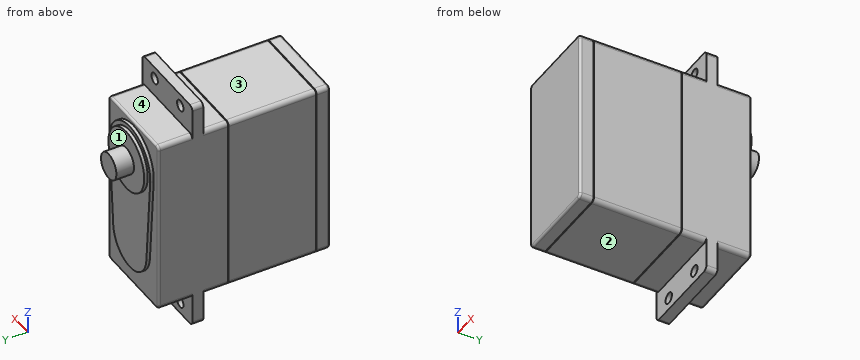
```python
from build123d import *

# Parameters (mm, degrees)
BOSS_EXTRU_1_DEPTH        = 9.75
BOSS_EXTRU_1_DEPTH_BACK   = 9.75
ESQUISSE1_W               = 40.5
ESQUISSE1_H               = 39
BOSS_EXTRU_2_DEPTH        = 0.8
CONG_6_R                  = 1
CONG_3_R                  = 0.5
ENL_V_MAT_EXTRU_3_DEPTH   = 0.2
ENL_V_MAT_EXTRU_2_DEPTH   = 0.2
BOSS_EXTRU_3_DEPTH        = 1.25
ENL_V_MAT_EXTRU_4_REACH   = 44.593
ESQUISSE10_R              = 1.25
SYM_TRIE3_COPY_1_REACH    = 44.593
SYM_TRIE3_COPY_1_SKETCH_R = 1.25


with BuildPart() as part:
    # Esquisse1 → Boss.-Extru.1 (new, two sides: drawn at the far end of the back side and taken through both)
    with BuildSketch(Plane(origin=(0, 0, 0), x_dir=(0, 0, -1), z_dir=(1, 0, 0)).offset(-BOSS_EXTRU_1_DEPTH_BACK)):
        Rectangle(ESQUISSE1_W, ESQUISSE1_H)
    extrude(amount=BOSS_EXTRU_1_DEPTH + BOSS_EXTRU_1_DEPTH_BACK)

    # Esquisse2 → Boss.-Extru.2 (add)
    with BuildSketch(Plane(origin=(13.65, 19.5, 0), x_dir=(0, 0, -1), z_dir=(0, 1, 0))):
        with BuildLine():
            Line((9.725609756, 20.13257629), (-10.664634146, 21.628555434))
            ThreePointArc((-10.664634146, 21.628555434), (-19.25, 13.65), (-10.664634146, 5.671444566))
            Line((-10.664634146, 5.671444566), (9.725609756, 7.16742371))
            ThreePointArc((9.725609756, 7.16742371), (15.75, 13.65), (9.725609756, 20.13257629))
        make_face()
    extrude(amount=BOSS_EXTRU_2_DEPTH)

    # Esquisse3 → R_volution1 (revolve)
    with BuildSketch(Plane(origin=(0, 0, 0), x_dir=(0, 0, -1), z_dir=(1, 0, 0)), mode=Mode.PRIVATE) as r_volution1_sk:
        Polygon((-4.25, 20.3), (-4.25, 21.1), (-8.25, 21.1), (-8.25, 25.1), (-11.25, 25.1), (-11.25, 20.3), align=None)
    revolve(r_volution1_sk.sketch.rotate(Axis((0, 19.890028941, 11.25), (0, -1, 0)), 180), axis=Axis((0, 19.890028941, 11.25), (0, -1, 0)))

    # Cong_6
    cong_6_edges = [part.edges().sort_by_distance(p)[0] for p in [
        (9.75, 0, 20.25),
        (-9.75, 0, -20.25),
        (9.75, 0, -20.25),
        (-9.75, 0, 20.25),
    ]]
    fillet(cong_6_edges, radius=CONG_6_R)

    # Cong_3
    cong_3_edges = [part.edges().sort_by_distance(p)[0] for p in [
        (0, 19.5, -20.25),
        (0, -19.5, -20.25),
        (0, 19.5, 20.25),
        (9.75, 19.5, 0),
        (-9.75, 19.5, 0),
        (-9.457106781, 19.5, 19.957106781),
        (9.457106781, 19.5, -19.957106781),
        (9.457106781, 19.5, 19.957106781),
        (-9.457106781, 19.5, -19.957106781),
        (-9.75, -19.5, 0),
        (9.75, -19.5, 0),
        (0, -19.5, 20.25),
        (-9.457106781, -19.5, 19.957106781),
        (9.457106781, -19.5, -19.957106781),
        (9.457106781, -19.5, 19.957106781),
        (-9.457106781, -19.5, -19.957106781),
    ]]
    fillet(cong_3_edges, radius=CONG_3_R)

    # Esquisse7 → Enl_v. mat.-Extru.3 (cut)
    with BuildSketch(Plane(origin=(0, -16.5, 0), x_dir=(-1, 0, 0), z_dir=(0, -1, 0))):
        with BuildLine():
            Line((8.75, -20.25), (-8.75, -20.25))
            ThreePointArc((-8.75, -20.25), (-9.457106781, -19.957106781), (-9.75, -19.25))
            Line((-9.75, -19.25), (-9.75, 19.25))
            ThreePointArc((-9.75, 19.25), (-9.457106781, 19.957106781), (-8.75, 20.25))
            Line((-8.75, 20.25), (8.75, 20.25))
            ThreePointArc((8.75, 20.25), (9.457106781, 19.957106781), (9.75, 19.25))
            Line((9.75, 19.25), (9.75, -19.25))
            ThreePointArc((9.75, -19.25), (9.457106781, -19.957106781), (8.75, -20.25))
        make_face()
        with BuildLine():
            Line((8.75, -20.05), (-8.75, -20.05))
            ThreePointArc((-8.75, -20.05), (-9.315685425, -19.815685425), (-9.55, -19.25))
            Line((-9.55, -19.25), (-9.55, 19.25))
            ThreePointArc((-9.55, 19.25), (-9.315685425, 19.815685425), (-8.75, 20.05))
            Line((-8.75, 20.05), (8.75, 20.05))
            ThreePointArc((8.75, 20.05), (9.315685425, 19.815685425), (9.55, 19.25))
            Line((9.55, 19.25), (9.55, -19.25))
            ThreePointArc((9.55, -19.25), (9.315685425, -19.815685425), (8.75, -20.05))
        make_face(mode=Mode.SUBTRACT)
    extrude(amount=-ENL_V_MAT_EXTRU_3_DEPTH, mode=Mode.SUBTRACT)

    # Esquisse6 → Enl_v. mat.-Extru.2 (cut)
    with BuildSketch(Plane(origin=(0, 3.5, 0), x_dir=(-1, 0, 0), z_dir=(0, -1, 0))):
        with BuildLine():
            Line((8.75, -20.25), (-8.75, -20.25))
            ThreePointArc((-8.75, -20.25), (-9.457106781, -19.957106781), (-9.75, -19.25))
            Line((-9.75, -19.25), (-9.75, 19.25))
            ThreePointArc((-9.75, 19.25), (-9.457106781, 19.957106781), (-8.75, 20.25))
            Line((-8.75, 20.25), (8.75, 20.25))
            ThreePointArc((8.75, 20.25), (9.457106781, 19.957106781), (9.75, 19.25))
            Line((9.75, 19.25), (9.75, -19.25))
            ThreePointArc((9.75, -19.25), (9.457106781, -19.957106781), (8.75, -20.25))
        make_face()
        with BuildLine():
            Line((8.75, -20.05), (-8.75, -20.05))
            ThreePointArc((-8.75, -20.05), (-9.315685425, -19.815685425), (-9.55, -19.25))
            Line((-9.55, -19.25), (-9.55, 19.25))
            ThreePointArc((-9.55, 19.25), (-9.315685425, 19.815685425), (-8.75, 20.05))
            Line((-8.75, 20.05), (8.75, 20.05))
            ThreePointArc((8.75, 20.05), (9.315685425, 19.815685425), (9.55, 19.25))
            Line((9.55, 19.25), (9.55, -19.25))
            ThreePointArc((9.55, -19.25), (9.315685425, -19.815685425), (8.75, -20.05))
        make_face(mode=Mode.SUBTRACT)
    extrude(amount=-ENL_V_MAT_EXTRU_2_DEPTH, mode=Mode.SUBTRACT)

    # Esquisse8 → Boss.-Extru.3 (add, symmetric)
    with BuildSketch(Plane(origin=(0, 10.5, 0), x_dir=(-1, 0, 0), z_dir=(0, -1, 0))):
        with BuildLine():
            Line((9.75, 19.25), (9.75, 26.25))
            ThreePointArc((9.75, 26.25), (9.457106781, 26.957106781), (8.75, 27.25))
            Line((8.75, 27.25), (-8.75, 27.25))
            ThreePointArc((-8.75, 27.25), (-9.457106781, 26.957106781), (-9.75, 26.25))
            Line((-9.75, 26.25), (-9.75, 19.25))
            ThreePointArc((-9.75, 19.25), (-9.457106781, 19.957106781), (-8.75, 20.25))
            Line((-8.75, 20.25), (8.75, 20.25))
            ThreePointArc((8.75, 20.25), (9.457106781, 19.957106781), (9.75, 19.25))
        make_face()
    boss_extru_3 = extrude(amount=BOSS_EXTRU_3_DEPTH, both=True)

    # Esquisse10 → Enl_v. mat.-Extru.4 (cut, up to next)
    with BuildSketch(Plane(origin=(0, 11.75, 0), x_dir=(1, 0, 0), z_dir=(0, 1, 0)), mode=Mode.PRIVATE) as enl_v_mat_extru_4_sk1:
        with Locations(Location((5, 24.5, 0), (0, 0, 270))):
            Circle(ESQUISSE10_R)
    enl_v_mat_extru_4_tool1 = extrude(enl_v_mat_extru_4_sk1.sketch, amount=-ENL_V_MAT_EXTRU_4_REACH, mode=Mode.PRIVATE) & part.part
    enl_v_mat_extru_4 = enl_v_mat_extru_4_tool1.solids().sort_by_distance((5, 11.75, -24.5))[0]
    add(enl_v_mat_extru_4, mode=Mode.SUBTRACT)

    # Sym_trie1: Boss.-Extru.3 across plane
    add(boss_extru_3.mirror(Plane.XY))

    # Sym_trie2: Enl_v. mat.-Extru.4 across plane
    add(enl_v_mat_extru_4.mirror(Plane(origin=(0, 0, 0), x_dir=(0, 0, 1), z_dir=(1, 0, 0))), mode=Mode.SUBTRACT)

    # Sym_trie3: Enl_v. mat.-Extru.4 across plane
    add(enl_v_mat_extru_4.mirror(Plane.XY), mode=Mode.SUBTRACT)

    # Sym_trie3 copy 1 sketch → Sym_trie3 copy 1 (cut, up to next)
    with BuildSketch(Plane(origin=(0, 11.75, 0), x_dir=(-1, 0, 0), z_dir=(0, 1, 0)), mode=Mode.PRIVATE) as sym_trie3_copy_1_sk1:
        with Locations(Location((5, 24.5, 0), (0, 0, 270))):
            Circle(SYM_TRIE3_COPY_1_SKETCH_R)
    sym_trie3_copy_1_tool1 = extrude(sym_trie3_copy_1_sk1.sketch, amount=-SYM_TRIE3_COPY_1_REACH, mode=Mode.PRIVATE) & part.part
    add(sym_trie3_copy_1_tool1.solids().sort_by_distance((-5, 11.75, 24.5))[0], mode=Mode.SUBTRACT)


solid = part.part
```
Geometry check sheet. Reference: the model listing, model coordinates, mm. Face numbers are marked on the shaded views. A direction names the side the tool comes from. Round coordinates to 2 decimals unless told otherwise and drop trailing zeros. Write each loop counter-clockwise with the first axis right and the second up, starting at its lowest first coordinate (ties: lowest second). Pieces come first, ordered by that corner, then holes. Notation, with made-up numbers: (73, 80) - (107, 80) arc R21 ccw to (107, 95) - close; hole circle Ø3 at (23, 38). An arc over 180 degrees is marked (long way). Write each question's results on one line, items separated by ' | '.
(1) Depth check by flat-ended pin: pin 1 Ø1.2 at (x, y) = (4.5, -18) entering from -Z; pin 2 Ø6 at (x, z) = (-0.5, 0.5) entering from +Y; pin 3 Ø4 at (x, z) = (-2.5, 24.5) entering from +Y. Enter the tip coordinate at first touch or a pass-through.
Computed:
pin 1: stops at z = -20.25 | pin 2: stops at y = 20.3 | pin 3: stops at y = 11.75
(2) Set-up check for the marked faces 1, 2, 3 and 4: record each of +Z, -Z, +X, -X, +Y, -Y from which the full face is reachable in a straight line by a thin tool's end or side.
Computed:
face 1: +Y | face 2: -Z, +X, -X, -Y | face 3: +Z, +X, -X, -Y | face 4: +Z, +X, -X, +Y
(3) Sectioned sample at C-C, the plane z = -5. Enter the section's corners in (x, y).
Computed:
outline: (-9.75, -19) arc R0.5 ccw to (-9.25, -19.5) - (9.25, -19.5) arc R0.5 ccw to (9.75, -19) - (9.75, -16.5) - (9.55, -16.5) - (9.55, -16.3) - (9.75, -16.3) - (9.75, 3.5) - (9.55, 3.5) - (9.55, 3.7) - (9.75, 3.7) - (9.75, 19) arc R0.5 ccw to (9.25, 19.5) - (6.83, 19.5) - (6.83, 20.3) - (-6.83, 20.3) - (-6.83, 19.5) - (-9.25, 19.5) arc R0.5 ccw to (-9.75, 19) - (-9.75, 3.7) - (-9.55, 3.7) - (-9.55, 3.5) - (-9.75, 3.5) - (-9.75, -16.3) - (-9.55, -16.3) - (-9.55, -16.5) - (-9.75, -16.5) - close
(4) Sectioned sample at B-B, the plane y = 7. Enter the section's corners in (x, z), plus the area to 3 significant figures.
Computed:
outline: (-9.75, -19.25) arc R1 ccw to (-8.75, -20.25) - (8.75, -20.25) arc R1 ccw to (9.75, -19.25) - (9.75, 19.25) arc R1 ccw to (8.75, 20.25) - (-8.75, 20.25) arc R1 ccw to (-9.75, 19.25) - close | area: 789 mm^2
(5) Sectioned sample at A-A, the plane z = 24.5. Enter the section's corners in (x, y), plus the area to 4 significant figures.
Computed:
outline: (-9.75, 9.25) - (-6.25, 9.25) - (-6.25, 11.75) - (-9.75, 11.75) - close; (-3.75, 9.25) - (3.75, 9.25) - (3.75, 11.75) - (-3.75, 11.75) - close; (6.25, 9.25) - (9.75, 9.25) - (9.75, 11.75) - (6.25, 11.75) - close | area: 36.25 mm^2
(6) Sectioned sample at D-D, the plane x = -5. Count the separate pieces of the cut face and the enclosed holes in it, plus the area to 3 significant figures.
Computed:
separate pieces: 3 | enclosed holes: 0 | area: 1,630 mm^2
(7) Thickness scan on probe 1 along Z at (x, y) = (-5, 9.9); probe 2 along X at (y, z) = (11.1, -24.5); probe 3 along Z at (x, y) = (-4, 10.5). Record the ranges inside material, lowest first. Write a range as from..to.
Computed:
probe 1: z = -27.25..-25.75, -23.25..23.25, 25.75..27.25 | probe 2: x = -9.75..-6.25, -3.75..3.75, 6.25..9.75 | probe 3: z = -27.25..-25.25, -23.75..23.75, 25.25..27.25
